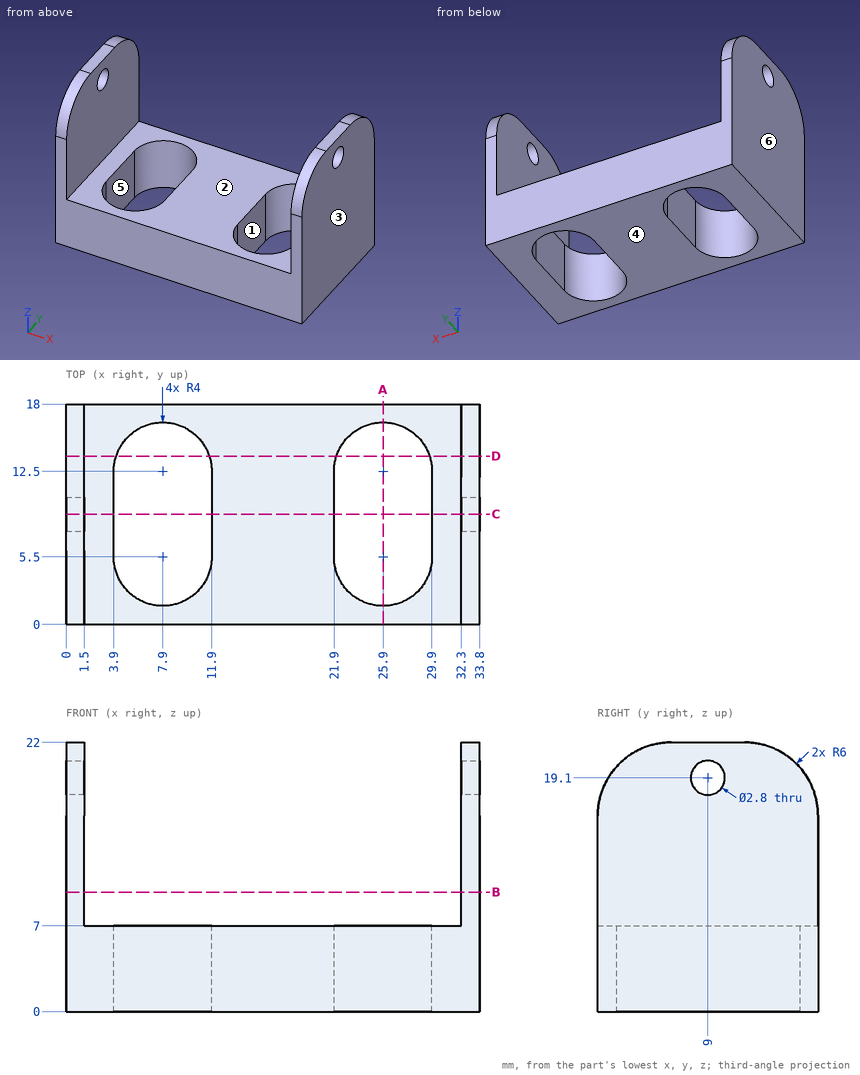
The figure shows three views and two pictorial views of one solid part (mm, origin at its lowest corner). Answer the questions. A direction names the side the tool comes from. Round coordinates to 2 decimals unless told otherwise and drop trailing zeros. Loops run counter-clockwise (first coordinate to the right, second up) from the corner with the lowest first, then second, coordinate; pieces in that order, holes last. Notation, with made-up numbers: (-9, 46) - (36, 46) arc R21 cw to (36, 79) - close; hole circle Ø11 at (-11, 61). An arc over 180 degrees is marked (long way). Use one line per item in the form item = value. Start each with the question number.
(1) Find section C-C on y = 9. Determine the outline of the cut face in (x, z), and give its area (3 significant figures).
(2) Determine the mould class of the marked faces 4, 5 and 6 for opening direction X: +X half, -X half, draft (parallel to the pull), parting line (faces both ways), or undercut.
(3) Consider line 1 (X direction, y = 7.5, z = 12.25); line 2 (X direction, y = 14.75, z = 4); line 3 (X direction, y = 2.75, z = 4.75). Determine where each line is inside the solid, lowest interval first.
(4) Find section B-B on z = 9.75. Determine the outline of the cut face in (x, y).
(5) Find section A-A on x = 25.9. Determine the outline of the cut face in (y, z), and give its area (3 significant figures).
(6) Which of the six approach directions +Z, -Z, +X, -X, +Y, -Y give full straight-line access (tool end or side, diameter ignored) to the marked faces 1, 2 and 3?
(7) Find section D-D on y = 13.75. Determine the outline of the cut face in (x, z).
Answer list:
q1.outline = (0, 0) - (3.9, 0) - (3.9, 7) - (1.5, 7) - (1.5, 17.7) - (0, 17.7) - close; (0, 20.5) - (1.5, 20.5) - (1.5, 22) - (0, 22) - close; (11.9, 0) - (21.9, 0) - (21.9, 7) - (11.9, 7) - close; (29.9, 0) - (33.8, 0) - (33.8, 17.7) - (32.3, 17.7) - (32.3, 7) - (29.9, 7) - close; (32.3, 20.5) - (33.8, 20.5) - (33.8, 22) - (32.3, 22) - close
q1.area = 161 mm^2
q2.face_4 = draft
q2.face_5 = undercut
q2.face_6 = -X half
q3.line_1 = 0 to 1.5, 32.3 to 33.8
q3.line_2 = 0 to 4.59, 11.21 to 22.59, 29.21 to 33.8
q3.line_3 = 0 to 5, 10.8 to 23, 28.8 to 33.8
q4.outline = (0, 0) - (1.5, 0) - (1.5, 18) - (0, 18) - close; (32.3, 0) - (33.8, 0) - (33.8, 18) - (32.3, 18) - close
q5.outline = (0, 0) - (1.5, 0) - (1.5, 7) - (0, 7) - close; (16.5, 0) - (18, 0) - (18, 7) - (16.5, 7) - close
q5.area = 21.0 mm^2
q6.face_1 = +Z, -Z
q6.face_2 = +Z, +Y, -Y
q6.face_3 = +Z, -Z, +X, +Y, -Y
q7.outline = (0, 0) - (4.1, 0) - (4.1, 7) - (1.5, 7) - (1.5, 21.74) - (0, 21.74) - close; (11.7, 0) - (22.1, 0) - (22.1, 7) - (11.7, 7) - close; (29.7, 0) - (33.8, 0) - (33.8, 21.74) - (32.3, 21.74) - (32.3, 7) - (29.7, 7) - close
